Geometry check sheet. Reference: the model listing, model coordinates, mm. A direction names the side the tool comes from. Give positions to 0.01 mm unless a question says otherwise; leave off trailing zeros. Loops run counter-clockwise (first coordinate to the right, second up) from the corner with the lowest first, then second, coordinate; pieces in that order, holes last. Notation, with made-up numbers: (65, 16) -> (106, 16) arc R18 cw to (106, 25) -> close; hole circle Ø6 at (31.25, 31.5). An arc over 180 degrees is marked (long way). One line per item, written item: value. Start each with the question number.
(1) Sectioned sample at A-A, the plane y = 365. Record the cut outline in (x, z).
(2) Gauge pin test, flat ends, axial feed: pin 1 Ø1 at (y, z) = (610, 1057) entering from +X; pin 2 Ø8 at (x, y) = (14, 512) entering from +Z. Record the tip position at first contact, or that the pin passes through.
(3) Sectioned sample at B-B, the plane x = 364. Record the cut outline in (y, z), then the cut area to 3 significant figures.
(4) Sectioned sample at C-C, the plane z = 412. Record the cut outline in (x, y), then the cut area to 3 significant figures.
(5) Scan lines: line 1 along X through (y, z) = (338, 1197.5); line 2 along Z through (x, y) = (559.5, 572.5). Record each from-to range of solid material in increasing order. Write a range as from..to.
(6) Tool access check on faces 1 (the face through (0, 592, 641)), 2 (the face through (272, 0, -2)). Record the directions out of +Z, -Z, +X, -X, +Y, -Y that give a thin tool (end or side, any length) a straight path to the whole face; none if there is none.
from build123d import *

# Parameters (mm, degrees)
F0_W     = 1200
F0_H     = 1200
F1_DEPTH = 200
F3_DEPTH = 1200


with BuildPart() as f1:
    # F0 (on Top) → F1 (new body)
    with BuildSketch(Plane.XY):
        with Locations((600, 600)):
            Rectangle(F0_W, F0_H)
    extrude(amount=-F1_DEPTH)

    # F2 (on face) → F3 (join)
    with BuildSketch(Plane.XZ):
        Polygon((-150, -200), (0, -200), (0, 0), (0, 1300), (-150, 1300), align=None)
    extrude(amount=-F3_DEPTH)


solid = f1.part
Calculated:
1. outline: (-150, -200) -> (1200, -200) -> (1200, 0) -> (0, 0) -> (0, 1300) -> (-150, 1300) -> close
2. pin 1: stops at x = 0
2. pin 2: stops at z = 0
3. outline: (0, -200) -> (1200, -200) -> (1200, 0) -> (0, 0) -> close
3. area: 240,000 mm2
4. outline: (-150, 0) -> (0, 0) -> (0, 1200) -> (-150, 1200) -> close
4. area: 180,000 mm2
5. line 1: x = -150..0
5. line 2: z = -200..0
6. face 1: +Z, +X, +Y, -Y
6. face 2: +Z, -Z, +X, -X, -Y
